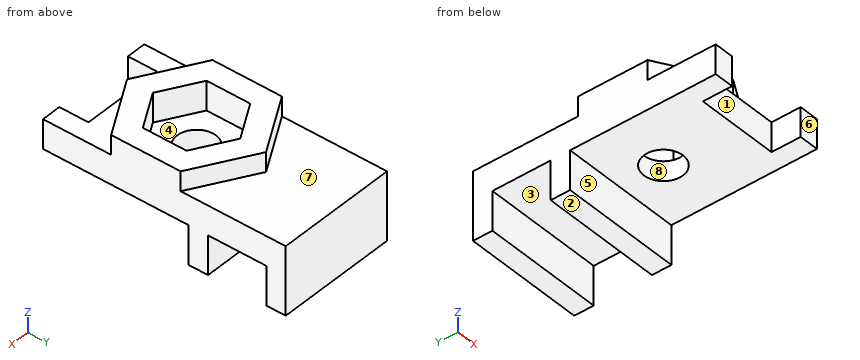
Solid Edge part; units mm, degrees
sketch "Sketch1" plane through (0, 0, 0) normal (0, 0, 1) x (1, 0, 0)
  line L0 (3.9, 2.5) -> (3.9, -7.5)
  line L1 (6.2, -7.5) -> (3.9, -7.5)
  line L2 (6.2, -12.5) -> (6.2, -7.5)
  line L3 (4.2, -12.5) -> (6.2, -12.5)
  line L4 (4.2, -9.5) -> (4.2, -12.5)
  line L5 (0, -9.5) -> (4.2, -9.5)
  line L6 (0, -9.5) -> (-4.2, -9.5)
  line L7 (-4.2, -9.5) -> (-4.2, -12.5)
  line L8 (-4.2, -12.5) -> (-6.2, -12.5)
  line L9 (-6.2, -12.5) -> (-6.2, -7.5)
  line L10 (-6.2, -7.5) -> (-3.9, -7.5)
  line L11 (-3.9, -7.5) -> (-3.9, 2.5)
  line L12 (-3.9, 2.5) -> (-3.9, 12.5)
  line L13 (-3.9, 12.5) -> (3.9, 12.5)
  line L14 (3.9, 12.5) -> (3.9, 2.5)
  circle A0 centre (0, -1.9) radius 2
extrude "Protrusion1" add sketch "Sketch1" along normal blind 3
sketch "Sketch2" plane through (0, 0, 0) normal (0, 0, -1) x (0, 1, 0)
  line L0 (12.5, -6.2) -> (-7.5, -6.2)
  line L1 (-7.5, -6.2) -> (-7.5, -3.9)
  line L2 (-7.5, -3.9) -> (7.5, -3.9)
  line L3 (7.5, -3.9) -> (7.5, 3.9)
  line L4 (7.5, 3.9) -> (-7.5, 3.9)
  line L5 (-7.5, 3.9) -> (-7.5, 6.2)
  line L6 (-7.5, 6.2) -> (12.5, 6.2)
  line L7 (12.5, 6.2) -> (12.5, -3.9)
  line L8 (12.5, -3.9) -> (12.5, -6.2)
extrude "Protrusion2" add sketch "Sketch2" against normal up to vertex (3 mm away)
sketch "Sketch3" plane through (0, 0, 3) normal (0, 0, 1) x (1, 0, 0)
  line L0 (0, 5.2591) -> (-6.2, 1.6796)
  line L1 (-6.2, 1.6796) -> (-6.2, -5.4796)
  line L2 (-6.2, -5.4796) -> (0, -9.0591)
  line L3 (0, -9.0591) -> (6.2, -5.4796)
  line L4 (6.2, -5.4796) -> (6.2, 1.6796)
  line L5 (6.2, 1.6796) -> (0, 5.2591)
  line L6 (0, 2.6033) -> (-3.9, 0.3517)
  line L7 (-3.9, 0.3517) -> (-3.9, -4.1517)
  line L8 (-3.9, -4.1517) -> (0, -6.4033)
  line L9 (0, -6.4033) -> (3.9, -4.1517)
  line L10 (3.9, -4.1517) -> (3.9, 0.3517)
  line L11 (3.9, 0.3517) -> (0, 2.6033)
extrude "ExtrudedProtrusion_3" add sketch "Sketch3" along normal blind 2
sketch "Sketch4" plane through (0, 0, 3) normal (0, 0, 1) x (1, 0, 0)
  line L0 (3.9, 0.3517) -> (0, 2.6033)
  line L1 (0, 2.6033) -> (-3.9, 0.3517)
  line L2 (-3.9, 0.3517) -> (-3.9, -4.1517)
  line L3 (-3.9, -4.1517) -> (0, -6.4033)
  line L4 (0, -6.4033) -> (3.9, -4.1517)
  line L5 (3.9, -4.1517) -> (3.9, 0.3517)
extrude "ExtrudedCutout_1" cut sketch "Sketch4" against normal blind 1
sketch "Sketch5" plane through (0, 0, 0) normal (0, 0, -1) x (-1, 0, 0)
  line L0 (6.2, 10.5) -> (-6.2, 10.5)
  line L1 (-6.2, 10.5) -> (-6.2, 12.5)
  line L2 (-6.2, 12.5) -> (6.2, 12.5)
  line L3 (6.2, 12.5) -> (6.2, 10.5)
  line L4 (6.2, 4.5) -> (-6.2, 4.5)
  line L5 (-6.2, 4.5) -> (-6.2, 2.5)
  line L6 (-6.2, 2.5) -> (6.2, 2.5)
  line L7 (6.2, 2.5) -> (6.2, 4.5)
extrude "ExtrudedProtrusion_4" add sketch "Sketch5" along normal blind 4
Geometry: final body of the model. Coordinates: model frame, mm. Face numbers are marked on the shaded views. A direction names the side the tool comes from. Round coordinates to 2 decimals unless told otherwise and drop trailing zeros. Order: outer loops, then holes, each group sorted by start corner. A loop starts at its lowest first (then second) coordinate and runs counter-clockwise, first axis right, second up. Notation, with made-up numbers: (69, 58) - (73, 58) arc R11 cw to (73, 70) - close; hole circle Ø11 at (33, 5.5). An arc over 180 degrees is marked (long way). Write item = value, one per line. Start each with the question number.
Q1. Cut plane C-C on x = 0.75. Return the cut outline in (y, z), and give its area (3 significant figures).
Q2. Access query for the marked faces 1, 2, 3, 4 and 5. Directions: +Z, -Z, +X, -X, +Y, -Y. A direction counts if a zero-diameter tool reaches every point of the face in a straight line with its end or side. Return the directions, or none.
Q3. Cut plane A-A on y = -1.9. Return the cut outline in (x, z).
Q4. Cut plane D-D on y = -10.75. Return the cut outline in (x, z).
Q5. Cut plane B-B on z = 0.75. Return the cut outline in (x, y).
Q6. Ray query, line 1 (Y direction, x = 0, z = 1.25); line 2 (X direction, y = -1.9, z = 0.65); line 3 (Y direction, x = -0.5, z = -0.75). Return the intervals inside material, ascending. Write a range as from..to.
Q7. Pin query (flat end, axial travel): pin 1 (1.2 mm diameter, centred on x = -2, z = -1, fed in from -Y); pin 2 (3.5 mm diameter, centred on x = -1.5, y = -5.5, fed in from -Z); pin 3 (2 mm diameter, centred on x = 2.5, y = 8, fed in from +Z). Return the tip coordinate at first contact, or that it passes through.
Q8. Pull-direction query (Y, two-part tool) for the marked faces 6, 7 and 8; classes: +Y half, -Y half, draft (parallel to the pull), parting line (faces both ways), or undercut.
Outcome:
q1.outline = (-9.5, 0) - (-3.75, 0) - (-3.75, 2) - (-5.97, 2) - (-5.97, 5) - (-8.63, 5) - (-8.63, 3) - (-9.5, 3) - close; (-0.05, 0) - (2.5, 0) - (2.5, -4) - (4.5, -4) - (4.5, 0) - (10.5, 0) - (10.5, -4) - (12.5, -4) - (12.5, 3) - (4.83, 3) - (4.83, 5) - (2.17, 5) - (2.17, 2) - (-0.05, 2) - close
q1.area = 77.1 mm^2
q2.face_1 = +Z, -Z, -Y
q2.face_2 = -Z, +X, -X, +Y, -Y
q2.face_3 = -Z, +X, -X
q2.face_4 = +Z
q2.face_5 = -Z, +X, -X, -Y
q3.outline = (-6.2, 0) - (-2, 0) - (-2, 2) - (-3.9, 2) - (-3.9, 5) - (-6.2, 5) - close; (2, 0) - (6.2, 0) - (6.2, 5) - (3.9, 5) - (3.9, 2) - (2, 2) - close
q4.outline = (-6.2, 0) - (-4.2, 0) - (-4.2, 3) - (-6.2, 3) - close; (4.2, 0) - (6.2, 0) - (6.2, 3) - (4.2, 3) - close
q5.outline = (-6.2, -12.5) - (-4.2, -12.5) - (-4.2, -9.5) - (4.2, -9.5) - (4.2, -12.5) - (6.2, -12.5) - (6.2, 12.5) - (-6.2, 12.5) - close; hole circle Ø4 at (0, -1.9)
q6.line_1 = -9.5..-3.9, 0.1..12.5
q6.line_2 = -6.2..-2, 2..6.2
q6.line_3 = 2.5..4.5, 10.5..12.5
q7.pin_1 = 2.5
q7.pin_2 = 0
q7.pin_3 = 3
q8.face_6 = -Y half
q8.face_7 = draft
q8.face_8 = undercut
